The drawing under review shows one solid part. Ordinate dimensions are in mm from its lowest x, y, z. A direction names the side the tool comes from. Coordinates: 2 decimals unless noted, no trailing zeros. Loops run counter-clockwise (first coordinate to the right, second up) from the corner with the lowest first, then second, coordinate; pieces in that order, holes last. Notation, with made-up numbers: M -6.5,-14.5 L 36.5,-14.5 A31 ccw 36.5,24.5 Z; hole C -2.5,36.5 d2. An arc over 180 degrees is marked long. Return JSON: item names as keys, results as strings.
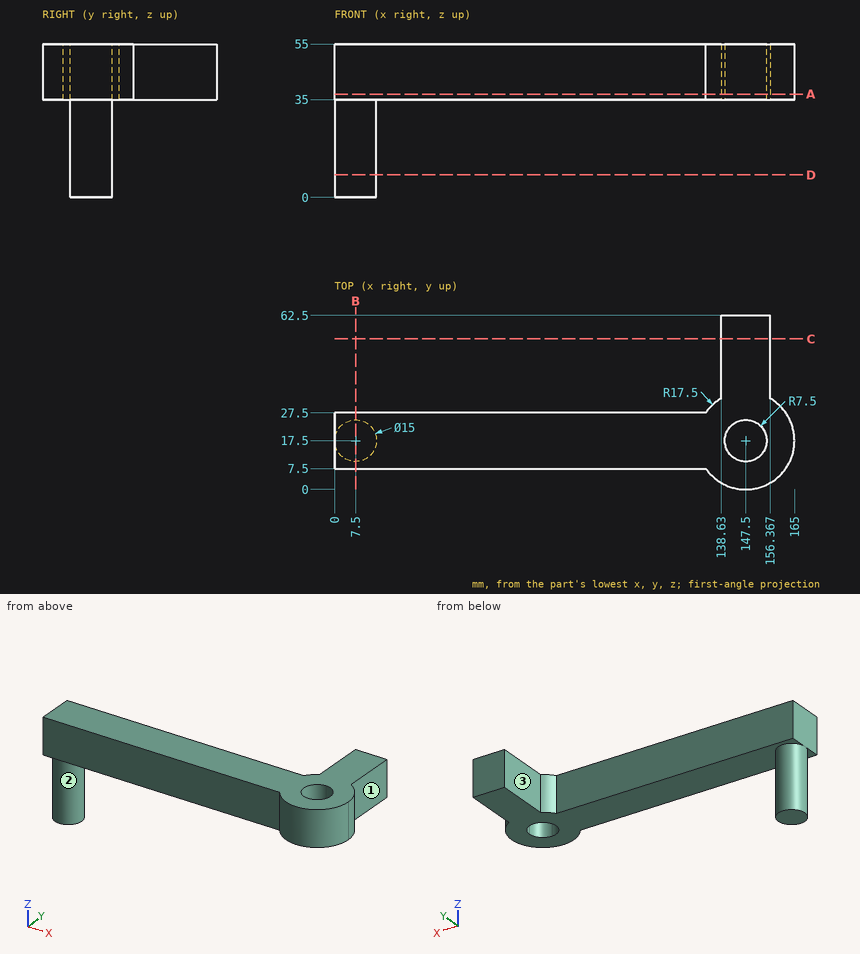
1. Add section B-B on x = 7.5. Give the boundary of the cut face in (y, z).
Check values:
{"outline": "M 7.5,35 L 10,35 L 10,0 L 25,0 L 25,35 L 27.5,35 L 27.5,55 L 7.5,55 Z"}
2. To check wall thickness, follow line 1 (X direction, y = 58, z = 45); line 2 (Z direction, x = 131.5, y = 16); line 3 (X direction, y = 23, z = 45) (1 decimal). State the ranges of each line that lie inside material, in increasing order.
Check values:
{"line 1": "138.63 to 156.37", "line 2": "35 to 55", "line 3": "0 to 142.4, 152.6 to 164.1"}
3. Add section A-A on z = 37. Give the boundary of the cut face in (x, y) (1 decimal), plus the area to 3 significant figures.
Check values:
{"outline": "M 0,7.5 L 133.1,7.5 A17.5 ccw long 156.4,32.6 L 156.4,62.5 L 138.6,62.5 L 138.6,32.6 A17.5 ccw 133.1,27.5 L 0,27.5 Z; hole C 147.5,17.5 d15", "area": "3,910 mm²"}
4. Add section C-C on y = 54. Give the boundary of the cut face in (x, z), plus the area to 3 significant figures.
Check values:
{"outline": "M 138.63,35 L 156.37,35 L 156.37,55 L 138.63,55 Z", "area": "355 mm²"}
5. Add section D-D on z = 8. Give the boundary of the cut face in (x, y).
Check values:
{"outline": "C 7.5,17.5 d15"}
6. Machinability: for the marked faces 1, 2 and 3, which of the approach directions +Z, -Z, +X, -X, +Y, -Y give a long, thin tool a straight path to every point of the face, cutting with its end or side? Answer none if there is none.
Check values:
{"face 1": "+Z, -Z, +X, +Y", "face 2": "-Z", "face 3": "+Z, -Z, -X, +Y"}
7. Insertion check: pin 1 Ø6 at (y, z) = (52, 44) entering from -X; pin 2 Ø1 at (x, y) = (141.5, 30) entering from -Z; pin 3 Ø16 at (y, z) = (42.5, 42) entering from +X. Each pin has a flat end and moves straight along its axis. Give the tip position at first contact, or say it passes through.
Check values:
{"pin 1": "x = 138.63", "pin 2": "z = 35", "pin 3": "x = 156.37"}
